Design review of the part built by this model. Coordinates are the model's own, in mm. A direction names the side the tool comes from. Round coordinates to 2 decimals unless told otherwise and drop trailing zeros. Write each loop counter-clockwise with the first axis right and the second up, starting at its lowest first coordinate (ties: lowest second). Pieces come first, ordered by that corner, then holes. Notation, with made-up numbers: M 72.5,-9 L 85.5,-9 A22 ccw 85.5,18 Z; hole C -35.75,9.25 d5. An arc over 180 degrees is marked long. Use CSV: the item, a comma, the result in double quotes.
from build123d import *

# Parameters (mm, degrees)
F0_R     = 38.1
F1_DEPTH = 12.7
F2_R     = 12.69999
F3_R     = 10.795
F4_DEPTH = 25.4
F6_R     = 12.065
F7_DEPTH = 6.35


# Not quite as in the source:
# - a fillet or chamfer is up to 0.001 mm smaller than in the source, because OpenCascade refuses the exact size


with BuildPart() as f1:
    # F0 (on Front) → F1 (new body)
    with BuildSketch(Plane.XZ):
        Circle(F0_R)
    extrude(amount=F1_DEPTH)

    # F2 (radius 12.7 in the source; OpenCascade refuses exactly that, so slightly less here)
    f2_edges = [f1.edges().sort_by_distance(p)[0] for p in [
        (-38.1, -12.7, 0),
    ]]
    fillet(f2_edges, radius=F2_R)

    # F3 (on Front) → F4 (cut)
    with BuildSketch(Plane.XZ):
        Circle(F3_R)
    extrude(amount=F4_DEPTH, mode=Mode.SUBTRACT)

    # F6 (on offset) → F7 (cut)
    with BuildSketch(Plane.XZ.offset(12.7)):
        Circle(F6_R)
    extrude(amount=-F7_DEPTH, mode=Mode.SUBTRACT)

    # F8: F1 across plane


with BuildPart() as f1_1:
    add(f1.part)
    add(f1.part.mirror(Plane.XZ))


solid = f1_1.part
1) For pin 1 Ø10 at (x, y) = (24.5, -8.5) entering from -Z; pin 2 Ø12 at (x, y) = (4, 0) entering from -Z; pin 3 Ø1 at (x, y) = (-24.5, 4.5) entering from +Z, all flat-tipped, find the tip position at first contact; note any pin that passes through.
Answers:
pin 1,"z = -30.63"
pin 2,"z = -38.1"
pin 3,"z = 28.59"
2) Add section C-C on y = -10.25. Write out the cut boundary in (x, z) (1 decimal).
Answers:
outline,"C 0,0 d65.8; hole C 0,0 d24.1"
3) The part is to be moulded in two halves that separate along X. For faces 4 (the face through (11.51, 9.57, 3.62)), 5 (the face through (11, 12.7, 6)), say which applies: released by +X, released by -X, zero draft, split by the parting line, or undercut.
Answers:
face 4,"undercut"
face 5,"zero draft"
4) Machinability: for faces 1 (the face through (11.51, -9.57, 3.62)), 2 (the face through (-2, 6.35, -11)), 3 (the face through (11, -12.7, 6)), which of the approach directions +Z, -Z, +X, -X, +Y, -Y give a long, thin tool a straight path to every point of the face, cutting with its end or side? Answer none if there is none.
Answers:
face 1,"-Y"
face 2,"+Y"
face 3,"+Z, -Z, +X, -X, -Y"
5) Wall thickness on line 1 along Z through (x, y) = (-1, 9.75); line 2 along Z through (x, y) = (0, 8.75) (3 decimals); line 3 along X through (y, z) = (7.5, 11): over which ranges is each line inside the solid? List them lowest first. Write a range as [from, to].
Answers:
line 1,"[-33.52, -12.02], [12.02, 33.52]"
line 2,"[-34.605, -12.065], [12.065, 34.605]"
line 3,"[-33.91, -4.96], [4.96, 33.91]"
6) Add section D-D on y = 7.75. Write out the cut boundary in (x, z) (3 decimals), then the cut area to 3 significant figures.
Answers:
outline,"C 0,0 d70.922; hole C 0,0 d24.13"
area,"3,490 mm²"
